Autodesk Inventor part; units mm, degrees
ref_plane "YZ Plane" through (0, 0, 0) normal (1, 0, 0) x (0, 1, 0)
ref_plane "XZ Plane" through (0, 0, 0) normal (0, 1, 0) x (-1, 0, 0)
ref_plane "XY Plane" through (0, 0, 0) normal (0, 0, 1) x (1, 0, 0)
sketch "Sketch1" plane through (0, 0, 0) normal (0, 1, 0) x (-1, 0, 0)
  line L0 (-6.35, 6.35) -> (6.35, 6.35)
  line L1 (6.35, 6.35) -> (6.35, -6.35)
  line L2 (6.35, -6.35) -> (-6.35, -6.35)
  line L3 (-6.35, -6.35) -> (-6.35, 6.35)
  line L4 (-6.35, 6.35) -> (6.35, -6.35) construction
  line L5 (6.35, 6.35) -> (-6.35, -6.35) construction
  point P0 (0, 0)
  dimension "d0" = 12.7
  dimension "d1" = 12.7
extrude "Extrusion1" add sketch "Sketch1" along normal blind 900
sketch "Sketch25" plane through (6.35, 0, 6.35) normal (0, 0, 1) x (1, 0, 0)
  circle A0 centre (-6.35, 875) radius 2.5
  line L0 (-12.7, 900) -> (0, 900)
  line L1 (0, 0) -> (0, 900)
  circle A1 centre (-6.35, 857) radius 2.5
  circle A2 centre (-6.35, 705) radius 2.5
  circle A3 centre (-6.35, 578) radius 2.5
  circle A4 centre (-6.35, 451) radius 2.5
  circle A5 centre (-6.35, 324) radius 2.5
  circle A6 centre (-6.35, 194) radius 2.5
  line L2 (0, 0) -> (-12.7, 0)
  point P0 (-6.35, 0)
  dimension "d197" = 5
  dimension "d198" = 25
  dimension "d199" = 6.35
  dimension "d200" = 5
  dimension "d201" = 18
  dimension "d202" = 6.35
  dimension "d210" = 5
  dimension "d211" = 152
  dimension "d212" = 6.35
  dimension "d213" = 5
  dimension "d214" = 127
  dimension "d215" = 5
  dimension "d216" = 127
  dimension "d217" = 5
  dimension "d218" = 127
  dimension "d219" = 5
  dimension "d220" = 130
hole "Hole23" at (0, 875, 6.35) at (0, 857, 6.35) at (0, 705, 6.35) at (0, 578, 6.35) at (0, 451, 6.35) at (0, 324, 6.35) at (0, 194, 6.35) direction (0, 0, -1) diameter 5 end through all
sketch "Sketch26" plane through (6.35, 0, -6.35) normal (1, 0, 0) x (0, 0, -1)
  circle A0 centre (-6.35, 883.5) radius 2.5
  line L0 (-12.7, 900) -> (0, 900)
  circle A1 centre (-6.35, 845.4) radius 2.5
  circle A2 centre (-6.35, 769.2) radius 2.5
  circle A3 centre (-6.35, 642.2) radius 2.5
  circle A4 centre (-6.35, 515.2) radius 2.5
  circle A5 centre (-6.35, 388.2) radius 2.5
  circle A6 centre (-6.35, 261.2) radius 2.5
  circle A7 centre (-6.35, 243.1152) radius 2.5
  circle A8 centre (-6.35, 217.7152) radius 2.5
  point P0 (-6.35, 0)
  dimension "d231" = 5
  dimension "d232" = 16.5
  dimension "d233" = 5
  dimension "d234" = 38.1
  dimension "d235" = 5
  dimension "d236" = 76.2
  dimension "d237" = 5
  dimension "d238" = 127
  dimension "d239" = 5
  dimension "d240" = 127
  dimension "d241" = 5
  dimension "d242" = 127
  dimension "d243" = 5
  dimension "d244" = 127
  dimension "d245" = 5
  dimension "d246" = 18.0848
  dimension "d247" = 5
  dimension "d248" = 25.4
hole "Hole24" at (6.35, 883.5, 0) at (6.35, 845.4, 0) at (6.35, 769.2, 0) at (6.35, 642.2, 0) at (6.35, 515.2, 0) at (6.35, 388.2, 0) at (6.35, 261.2, 0) at (6.35, 243.1152, 0) at (6.35, 217.7152, 0) direction (-1, 0, 0) diameter 5 end through all
thread "Thread1"
thread "Thread2"
thread "Thread3"
thread "Thread4"
thread "Thread5"
thread "Thread6"
thread "Thread7"
thread "Thread8"
thread "Thread9"
thread "Thread10"
properties part number "Rod"
Work out the finished part from the listing and answer in its coordinate system (mm). Round coordinates to 2 decimals unless told otherwise and drop trailing zeros. Write each question's results on one line, items separated by ' | '. Start each with the question number.
1. Given pin 1 Ø4.5 at (y, z) = (515.2, 0) entering from -X, flat-ended and moving along its own axis, determine where the tip first touches the part or whether it passes through.
2. Section A-A (x = 0) is taken. State how many separate pieces and enclosed holes the cut face has, plus the area to 3 significant figures.
3. Find the intervals of material crossed by probe 1 along Z at (x, y) = (0.75, 388.2); probe 2 along X at (y, z) = (452, -0.25), in increasing order. Write a range as from..to.
Evaluation:
1) pin 1: passes through
2) separate pieces: 8 | enclosed holes: 9 | area: 10,800 mm2
3) probe 1: z = -6.35..-2.5, 2.5..6.35 | probe 2: x = -6.35..-2.29, 2.29..6.35
